```python
from build123d import *

# Parameters (mm, degrees)
SKETCH1_W             = 22
SKETCH1_H             = 2
BOSS_EXTRUDE1_DEPTH   = 10
BOSS_EXTRUDE1_2_DEPTH = 10
SKETCH1_H_2           = 12
BOSS_EXTRUDE1_3_DEPTH = 10
SKETCH1_W_2           = 44
BOSS_EXTRUDE1_4_DEPTH = 10
SKETCH1_W_3           = 120
SKETCH1_H_3           = 10.5
SKETCH1_R             = 3
BOSS_EXTRUDE1_5_DEPTH = 10
BOSS_EXTRUDE1_6_DEPTH = 10
SKETCH1_5_W           = 6
SKETCH1_5_H           = 20
BOSS_EXTRUDE2_DEPTH   = 25
BOSS_EXTRUDE3_DEPTH   = 4
SKETCH1_8_R           = 3
SKETCH1_8_R_2         = 1.5
BOSS_EXTRUDE4_DEPTH   = 10
SKETCH1_10_R          = 3
SKETCH1_10_R_2        = 1.5
CUT_EXTRUDE1_DEPTH    = 4
SKETCH3_R             = 1.5
CUT_EXTRUDE4_DEPTH    = 14
SKETCH4_R             = 1.5
CUT_EXTRUDE5_DEPTH    = 14
CUT_EXTRUDE6_DEPTH    = 59
SKETCH5_4_W           = 3.2
SKETCH5_4_H           = 6.2
CUT_EXTRUDE8_DEPTH    = 59
SKETCH1_11_R          = 1.5
CUT_EXTRUDE9_DEPTH    = 59
SKETCH6_W             = 2.316345527
SKETCH6_H             = 6
CUT_EXTRUDE10_DEPTH   = 13
FILLET1_R             = 8
SKETCH7_R             = 0.85
CUT_EXTRUDE13_DEPTH   = 6


with BuildPart() as part:
    # Sketch1 → Boss-Extrude1 (new body)
    with BuildSketch(Plane.XY):
        with Locations((21.319715808, 11)):
            Rectangle(SKETCH1_W, SKETCH1_H)
    extrude(amount=BOSS_EXTRUDE1_DEPTH)



with BuildPart() as body_2:
    # Sketch1 → Boss-Extrude1 2 (new body)
    with BuildSketch(Plane.XY):
        with Locations((21.319715808, 1)):
            Rectangle(SKETCH1_W, SKETCH1_H)
    extrude(amount=BOSS_EXTRUDE1_2_DEPTH)


with BuildPart() as body_3:
    # Sketch1 → Boss-Extrude1 3 (new body)
    with BuildSketch(Plane.XY):
        with Locations((49.319715808, 6)):
            Rectangle(SKETCH1_W, SKETCH1_H_2)
    extrude(amount=BOSS_EXTRUDE1_3_DEPTH)


with BuildPart() as body_4:
    # Sketch1 → Boss-Extrude1 4 (new body)
    with BuildSketch(Plane.XY):
        with Locations((-37.680284192, 6)):
            Rectangle(SKETCH1_W_2, SKETCH1_H_2)
    extrude(amount=BOSS_EXTRUDE1_4_DEPTH)


with BuildPart() as body_5:
    # Sketch1 → Boss-Extrude1 5 (new body)
    with BuildSketch(Plane.XY):
        with Locations((0.319715808, -18.75)):
            Rectangle(SKETCH1_W_3, SKETCH1_H_3)
        with Locations((-55.180284192, -19.5)):
            Circle(SKETCH1_R, mode=Mode.SUBTRACT)
        with Locations((55.819715808, -19.5)):
            Circle(SKETCH1_R, mode=Mode.SUBTRACT)
    extrude(amount=BOSS_EXTRUDE1_5_DEPTH)


with BuildPart() as body_6:
    # Sketch1 → Boss-Extrude1 6 (new body)
    with BuildSketch(Plane.XY):
        with Locations((0.319715808, 30.75)):
            Rectangle(SKETCH1_W_3, SKETCH1_H_3)
        with Locations((-55.180284192, 31.5)):
            Circle(SKETCH1_R, mode=Mode.SUBTRACT)
        with Locations((55.819715808, 31.5)):
            Circle(SKETCH1_R, mode=Mode.SUBTRACT)
    extrude(amount=BOSS_EXTRUDE1_6_DEPTH)


with BuildPart() as part_1:
    add(part.part)

    add(body_2.part)  # Boss-Extrude2 merges body 2

    add(body_3.part)  # Boss-Extrude2 merges body 3

    add(body_4.part)  # Boss-Extrude2 merges body 4
    # Sketch1_5 → Boss-Extrude2 (add)
    with BuildSketch(Plane.XY):
        with Locations((-12.680284192, 6)):
            Rectangle(SKETCH1_5_W, SKETCH1_5_H)
        Polygon((38.319715808, 0), (38.319715808, 12), (38.319715808, 15.500704621), (38.319715808, 16), (32.319715808, 16), (32.319715808, 15.500704621), (32.319715808, 12), (32.319715808, 10), (32.319715808, 2), (32.319715808, 0), (32.319715808, -3.500704621), (32.319715808, -4), (38.319715808, -4), (38.319715808, -3.500704621), align=None)
    extrude(amount=BOSS_EXTRUDE2_DEPTH)


    add(body_5.part)  # Boss-Extrude3 merges body 5

    add(body_6.part)  # Boss-Extrude3 merges body 6
    # Sketch1_6 → Boss-Extrude3 (add)
    # profile 1 of 3: a face of its own
    with BuildSketch(Plane.XY):
        Polygon((-15.680284192, 0), (-59.680284192, 0), (-59.680284192, -13.5), (60.319715808, -13.5), (60.319715808, 0), (38.319715808, 0), (38.319715808, -3.500704621), (38.319715808, -4), (32.319715808, -4), (32.319715808, -3.500704621), (32.319715808, 0), (10.319715808, 0), (-9.680284192, 0), (-9.680284192, -4), (-15.680284192, -4), align=None)
        with BuildLine():
            Line((38.319715808, -11.5), (-37.680284192, -11.5))
            ThreePointArc((-37.680284192, -11.5), (-39.930284192, -9.25), (-37.680284192, -7))
            Line((-37.680284192, -7), (38.319715808, -7))
            ThreePointArc((38.319715808, -7), (40.569715808, -9.25), (38.319715808, -11.5))
        make_face(mode=Mode.SUBTRACT)
    # profile 2 of 3: a face of its own
    with BuildSketch(Plane.XY):
        Polygon((60.319715808, 25.5), (-59.680284192, 25.5), (-59.680284192, 12), (-15.680284192, 12), (-15.680284192, 16), (-9.680284192, 16), (-9.680284192, 12), (10.319715808, 12), (32.319715808, 12), (32.319715808, 15.500704621), (32.319715808, 16), (38.319715808, 16), (38.319715808, 15.500704621), (38.319715808, 12), (60.319715808, 12), align=None)
        with BuildLine():
            ThreePointArc((-37.680284192, 19), (-39.930284192, 21.25), (-37.680284192, 23.5))
            Line((-37.680284192, 23.5), (38.319715808, 23.5))
            ThreePointArc((38.319715808, 23.5), (40.569715808, 21.25), (38.319715808, 19))
            Line((38.319715808, 19), (-37.680284192, 19))
        make_face(mode=Mode.SUBTRACT)
    # profile 3 of 3: a face of its own
    with BuildSketch(Plane.XY):
        Polygon((10.319715808, 12), (-9.680284192, 12), (-9.680284192, 0), (10.319715808, 0), (10.319715808, 2), (32.319715808, 2), (32.319715808, 10), (10.319715808, 10), align=None)
    extrude(amount=BOSS_EXTRUDE3_DEPTH)

    # Sketch1_8 → Boss-Extrude4 (add)
    # profile 1 of 4: a face of its own
    with BuildSketch(Plane.XY):
        with Locations((-55.180284192, 31.5)):
            Circle(SKETCH1_8_R)
        with Locations((-55.180284192, 31.5)):
            Circle(SKETCH1_8_R_2, mode=Mode.SUBTRACT)
    # profile 2 of 4: a face of its own
    with BuildSketch(Plane.XY):
        with Locations((-55.180284192, -19.5)):
            Circle(SKETCH1_8_R)
        with Locations((-55.180284192, -19.5)):
            Circle(SKETCH1_8_R_2, mode=Mode.SUBTRACT)
    # profile 3 of 4: a face of its own
    with BuildSketch(Plane.XY):
        with Locations((55.819715808, -19.5)):
            Circle(SKETCH1_8_R)
        with Locations((55.819715808, -19.5)):
            Circle(SKETCH1_8_R_2, mode=Mode.SUBTRACT)
    # profile 4 of 4: a face of its own
    with BuildSketch(Plane.XY):
        with Locations((55.819715808, 31.5)):
            Circle(SKETCH1_8_R)
    extrude(amount=BOSS_EXTRUDE4_DEPTH)

    # Sketch1_10 → Cut-Extrude1 (cut)
    # profile 1 of 4: a face of its own
    with BuildSketch(Plane.XY):
        with Locations((55.819715808, 31.5)):
            Circle(SKETCH1_10_R)
        with Locations((55.819715808, 31.5)):
            Circle(SKETCH1_10_R_2, mode=Mode.SUBTRACT)
    # profile 2 of 4: a face of its own
    with BuildSketch(Plane.XY):
        with Locations((55.819715808, -19.5)):
            Circle(SKETCH1_10_R)
        with Locations((55.819715808, -19.5)):
            Circle(SKETCH1_10_R_2, mode=Mode.SUBTRACT)
    # profile 3 of 4: a face of its own
    with BuildSketch(Plane.XY):
        with Locations((-55.180284192, -19.5)):
            Circle(SKETCH1_10_R)
        with Locations((-55.180284192, -19.5)):
            Circle(SKETCH1_10_R_2, mode=Mode.SUBTRACT)
    # profile 4 of 4: a face of its own
    with BuildSketch(Plane.XY):
        with Locations((-55.180284192, 31.5)):
            Circle(SKETCH1_10_R)
        with Locations((-55.180284192, 31.5)):
            Circle(SKETCH1_10_R_2, mode=Mode.SUBTRACT)
    extrude(amount=CUT_EXTRUDE1_DEPTH, mode=Mode.SUBTRACT)

    # Sketch3 → Cut-Extrude4 (cut)
    with BuildSketch(Plane.XY.offset(25)):
        with Locations((-12.680284192, 11)):
            Circle(SKETCH3_R)
        with Locations((-12.680284192, 1)):
            Circle(SKETCH3_R)
    extrude(amount=-CUT_EXTRUDE4_DEPTH, mode=Mode.SUBTRACT)

    # Sketch4 → Cut-Extrude5 (cut)
    with BuildSketch(Plane.XY.offset(25)):
        with Locations((35.319715808, 10.999295379)):
            Circle(SKETCH4_R)
        with Locations((35.319715808, 0.999295379)):
            Circle(SKETCH4_R)
    extrude(amount=-CUT_EXTRUDE5_DEPTH, mode=Mode.SUBTRACT)

    # Sketch5 → Cut-Extrude6 (cut)
    with BuildSketch(Plane.ZY.offset(15.680284192)):
        Polygon((10, 12), (15, 16), (4, 16), (4, 12), align=None)
        Polygon((4, -4), (15, -4), (10, 0), (4, 0), align=None)
    extrude(amount=-CUT_EXTRUDE6_DEPTH, mode=Mode.SUBTRACT)

    # Sketch5_4 → Cut-Extrude8 (cut)
    with BuildSketch(Plane.ZY.offset(15.680284192)):
        with Locations((17.706989835, 0.475595868)):
            Rectangle(SKETCH5_4_W, SKETCH5_4_H)
        with Locations((17.409200428, 10.831284061)):
            Rectangle(SKETCH5_4_W, SKETCH5_4_H)
    extrude(amount=-CUT_EXTRUDE8_DEPTH, mode=Mode.SUBTRACT)

    # Sketch1_11 → Cut-Extrude9 (cut)
    with BuildSketch(Plane.XY):
        with Locations((55.819715808, 31.5)):
            Circle(SKETCH1_11_R)
    extrude(amount=CUT_EXTRUDE9_DEPTH, mode=Mode.SUBTRACT)

    # Sketch6 → Cut-Extrude10 (cut)
    with BuildSketch(Plane(origin=(0, 0, 0), x_dir=(-1, 0, 0), z_dir=(0, -1, 0))):
        with Locations((-11.477888571, -7)):
            Rectangle(SKETCH6_W, SKETCH6_H)
    extrude(amount=-CUT_EXTRUDE10_DEPTH, mode=Mode.SUBTRACT)

    # Fillet1
    fillet1_edges = [part_1.edges().sort_by_distance(p)[0] for p in [
        (60.319715808, -24, 5),
        (-59.680284192, -24, 5),
        (60.319715808, 36, 5),
        (-59.680284192, 36, 5),
    ]]
    fillet(fillet1_edges, radius=FILLET1_R)

    # Sketch7 → Cut-Extrude13 (cut)
    with BuildSketch(Plane(origin=(0, 0, 0), x_dir=(-1, 0, 0), z_dir=(0, 0, -1))):
        with Locations((51.035618514, 33.268406719)):
            Circle(SKETCH7_R)
        with Locations((45.535618514, 32.990148628)):
            Circle(SKETCH7_R)
        with Locations((56.409164496, 27.113974119)):
            Circle(SKETCH7_R)
        with Locations((-46.279640328, -21.012456623)):
            Circle(SKETCH7_R)
        with Locations((-51.779640328, -21.290714713)):
            Circle(SKETCH7_R)
        with Locations((-57.153186309, -15.136282114)):
            Circle(SKETCH7_R)
        with Locations((45.535618514, 27.113974119)):
            Circle(SKETCH7_R)
        with Locations((-46.279640328, -15.136282114)):
            Circle(SKETCH7_R)
    extrude(amount=-CUT_EXTRUDE13_DEPTH, mode=Mode.SUBTRACT)


solid = part_1.part
```
Could you check a few things on this model? Use its own coordinates, in mm. A direction names the side the tool comes from. Round coordinates to 2 decimals unless told otherwise and drop trailing zeros. Write each loop counter-clockwise with the first axis right and the second up, starting at its lowest first coordinate (ties: lowest second). Pieces come first, ordered by that corner, then holes.
(1) Suppose I cut it at C-C on x = -36.5. Write out the boundary of the cut face in (y, z).
Findings below:
outline: (-24, 0) - (-11.5, 0) - (-11.5, 4) - (-13.5, 4) - (-13.5, 10) - (-24, 10) - close; (-7, 0) - (19, 0) - (19, 4) - (12, 4) - (12, 10) - (0, 10) - (0, 4) - (-7, 4) - close; (23.5, 0) - (36, 0) - (36, 10) - (25.5, 10) - (25.5, 4) - (23.5, 4) - close
(2) Suppose I cut it at A-A on x = 4.5. Write out the boundary of the cut face in (y, z), and give its area (3 significant figures).
Findings below:
outline: (-24, 0) - (-11.5, 0) - (-11.5, 4) - (-13.5, 4) - (-13.5, 10) - (-24, 10) - close; (-7, 0) - (19, 0) - (19, 4) - (-7, 4) - close; (23.5, 0) - (36, 0) - (36, 10) - (25.5, 10) - (25.5, 4) - (23.5, 4) - close
area: 330 mm2
(3) For pin 1 (5 mm diameter, centred on x = -13.5, z = 19, fed in from +Y); pin 2 (0.9 mm diameter, centred on x = 52, y = -21, fed in from -Z); pin 3 (4 mm diameter, centred on x = 55.82, y = 31.5, fed in from -Z), each with a flat end and sliding along its axis, tell me the tip position at first contact or that it passes through.
Findings below:
pin 1: stops at y = 16
pin 2: stops at z = 6
pin 3: stops at z = 4
(4) If I drill on probe 1 along Y at (x, z) = (20, 1); probe 2 along Y at (x, z) = (17.5, 8.75); probe 3 along X at (y, z) = (14, 17.5), over which ranges is the centre line in solid material (lowest first)?
Findings below:
probe 1: y = -24 to -11.5, -7 to 19, 23.5 to 36
probe 2: y = -24 to -13.5, 0 to 2, 10 to 12, 25.5 to 36
probe 3: x = -15.68 to -9.68, 32.32 to 38.32
(5) Suppose I cut it at D-D on x = 44. Write out the boundary of the cut face in (y, z), and give its area (3 significant figures).
Findings below:
outline: (-24, 0) - (36, 0) - (36, 10) - (25.5, 10) - (25.5, 4) - (12, 4) - (12, 10) - (0, 10) - (0, 4) - (-13.5, 4) - (-13.5, 10) - (-24, 10) - close
area: 438 mm2
(6) Suppose I cut it at B-B on y = 21.25. Write out the boundary of the cut face in (x, z).
Findings below:
outline: (-59.68, 0) - (-39.93, 0) - (-39.93, 4) - (-59.68, 4) - close; (40.57, 0) - (60.32, 0) - (60.32, 4) - (40.57, 4) - close
(7) Thinking about a two-plate mould opening in X: for faces 5 (the face through (38.32, 6, 17)), 6 (the face through (-56.3, -18.5, 7)), 7 (the face through (-12.7, 14, 12.5)), which applies, +X half, -X half, draft (parallel to the pull), parting line (faces both ways), or undercut?
Findings below:
face 5: +X half
face 6: undercut
face 7: draft
(8) Which directions (+Z, -Z, +X, -X, +Y, -Y) give clear straight access to the entire face, cutting with the end or side of a thin tool? Please do faces 1 (the face through (40.57, 21.3, 1.97)), 2 (the face through (22, 10, 7)), 3 (the face through (49, 6, 10)), 4 (the face through (35, 3.576, 18)).
Findings below:
face 1: +Z, -Z
face 2: +Z
face 3: +Z, +X, +Y, -Y
face 4: +X, -X
